Design review of the part shown in the three views and the two pictorial views. Dimensions are in mm from the part's minimum x, y and z. Give positions to 0.01 mm unless a question says otherwise; leave off trailing zeros. Order: outer loops, then holes, each group sorted by start corner. A loop starts at its lowest first (then second) coordinate and runs counter-clockwise, first axis right, second up. Notation, with made-up numbers: (-28.75, 57.25) -> (-17.75, 57.25) arc R15 cw to (-17.75, 73.25) -> close; hole circle Ø4 at (-1.5, 4). An arc over 180 degrees is marked (long way). Use one line per item in the form item = value.
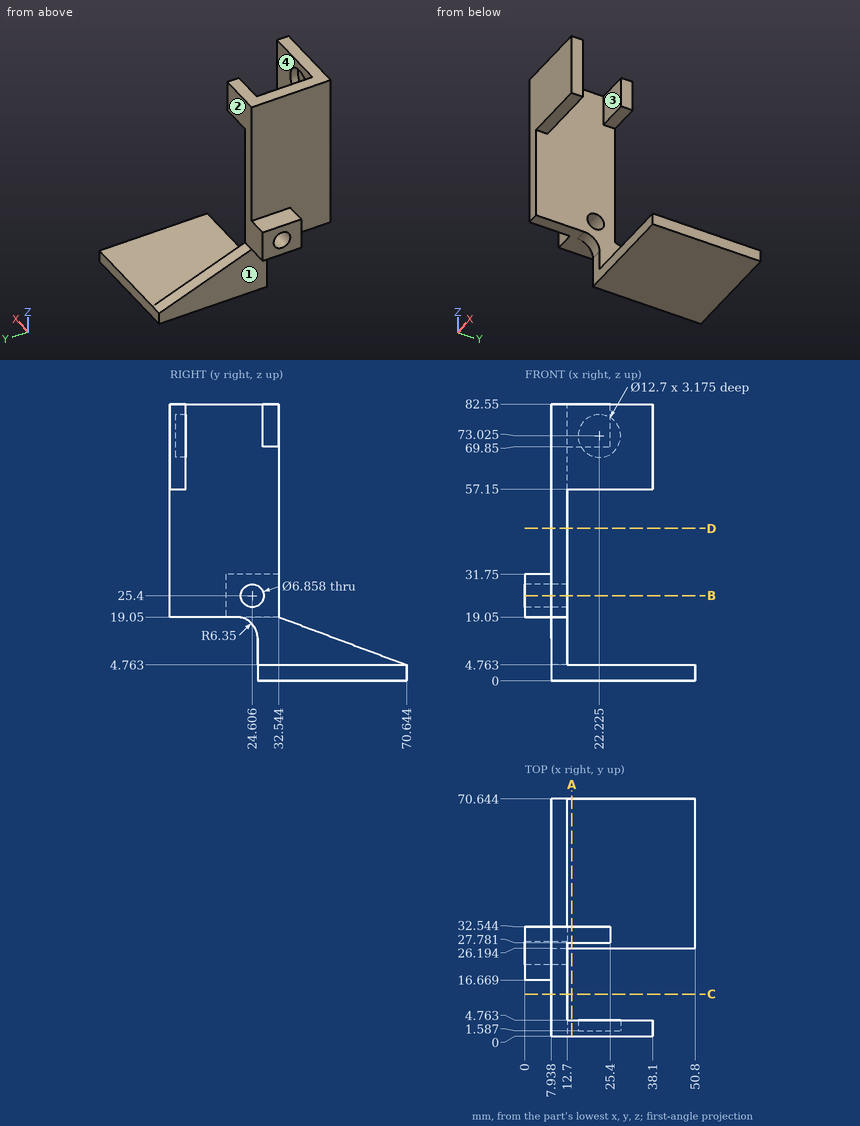
1. For L1, parallel to Z at x = 13.5, y = 31; L2, parallel to Y at x = 9, z = 25.4 (1 decimal); L3, parallel to Y at x = 7.5, z = 25.4 (1 decimal), list the stretches that pass through material, from the lowest coordinate up.
Values:
L1 = 0 to 4.76, 69.85 to 82.55
L2 = 0 to 21.2, 28 to 32.5
L3 = 16.7 to 21.2, 28 to 32.5
2. Add section C-C on y = 12.5. Give the boundary of the cut face in (x, z).
Values:
outline = (7.94, 19.05) -> (12.7, 19.05) -> (12.7, 82.55) -> (7.94, 82.55) -> close
3. Add section A-A on x = 14. Give the boundary of the cut face in (y, z), then the cut area to 3 significant figures.
Values:
outline = (0, 57.15) -> (4.76, 57.15) -> (4.76, 82.55) -> (0, 82.55) -> close; (26.19, 0) -> (70.64, 0) -> (70.64, 4.76) -> (26.19, 4.76) -> close; (27.78, 69.85) -> (32.54, 69.85) -> (32.54, 82.55) -> (27.78, 82.55) -> close
area = 393 mm^2
4. Add section B-B on z = 25.4. Give the boundary of the cut face in (x, y) (1 decimal), then the cut area to 3 significant figures.
Values:
outline = (0, 16.7) -> (7.9, 16.7) -> (7.9, 0) -> (12.7, 0) -> (12.7, 21.2) -> (0, 21.2) -> close; (0, 28) -> (12.7, 28) -> (12.7, 32.5) -> (0, 32.5) -> close
area = 194 mm^2
5. Add section D-D on z = 45.5. Give the boundary of the cut face in (x, y).
Values:
outline = (7.94, 0) -> (12.7, 0) -> (12.7, 32.54) -> (7.94, 32.54) -> close
6. For pin 1 Ø5.5 at (y, z) = (53.5, 13) entering from -X; pin 2 Ø4 at (x, y) = (5, 23.5) entering from +Z; pin 3 Ø2.5 at (x, z) = (3.5, 27) entering from -Y, all flat-tipped, find the tip position at first contact; note any pin that passes through.
Values:
pin_1 = 7.94
pin_2 = 31.75
pin_3 = 16.67
7. The part is to be moulded in two halves that separate along Y. For the marked faces 1, 2, 3 and 4, say which applies: +Y half, -Y half, draft (parallel to the pull), parting line (faces both ways), or undercut.
Values:
face_1 = draft
face_2 = +Y half
face_3 = undercut
face_4 = undercut
